Autodesk Inventor part; units mm, degrees
ref_plane "YZ Plane" through (0, 0, 0) normal (1, 0, 0) x (0, 1, 0)
ref_plane "XZ Plane" through (0, 0, 0) normal (0, 1, 0) x (-1, 0, 0)
ref_plane "XY Plane" through (0, 0, 0) normal (0, 0, 1) x (1, 0, 0)
sketch "Sketch1" plane through (0, 0, 0) normal (0, 1, 0) x (-1, 0, 0)
  arc A0 (24.9, 14.1574) -> (29.1, 14.1574) centre (27, 14.1574) ccw
  line L0 (29.1, 14.1574) -> (29.1, 29.1574)
  arc A1 (29.1, 29.1574) -> (24.9, 29.1574) centre (27, 29.1574) ccw
  line L1 (24.9, 29.1574) -> (24.9, 14.1574)
  arc A2 (-29.1, 14.1574) -> (-24.9, 14.1574) centre (-27, 14.1574) ccw
  line L2 (-24.9, 14.1574) -> (-24.9, 29.1574)
  arc A3 (-24.9, 29.1574) -> (-29.1, 29.1574) centre (-27, 29.1574) ccw
  line L3 (-29.1, 29.1574) -> (-29.1, 14.1574)
  ellipse E0 centre (7.3196, 102.715) end of major axis (13.9835, 105.6762) minor radius 6.4402 (10.2387, 108.9524) -> (7.9784, 109.3033) ccw
  line L4 (7.9784, 109.3033) -> (-7.9784, 109.3033)
  ellipse E1 centre (-7.3196, 102.715) end of major axis (-0.6557, 99.7539) minor radius 6.4402 (-7.9784, 109.3033) -> (-10.2387, 108.9524) ccw
  arc A4 (-14.0587, 108.0035) -> (-10.2387, 108.9524) centre (-18.8823, 135.5849) ccw
  arc A5 (-14.0587, 108.0035) -> (-17.7444, 104.1628) centre (-13.2835, 103.5708) ccw
  arc A6 (-18.815, 99.3694) -> (-17.7444, 104.1628) centre (-45.5011, 107.8461) ccw
  line L5 (-18.815, 99.3694) -> (-24.7592, 80.6562)
  arc A7 (-24.7592, 80.6562) -> (-24.9, 79.748) centre (-21.9, 79.748) ccw
  line L6 (-24.9, 79.748) -> (-24.9, 68.8185)
  arc A8 (-27.8412, 67.0538) -> (-24.9, 68.8185) centre (-26.9, 68.8185) ccw
  arc A9 (-27.8412, 67.0538) -> (-30.3028, 66.5886) centre (-28.7824, 65.2891) ccw
  arc A10 (-34.9925, 63.1171) -> (-30.3028, 66.5886) centre (-40.1848, 75.0352) ccw
  arc A11 (-34.9925, 63.1171) -> (-38.8388, 42.8186) centre (-30, 51.6574) ccw
  line L7 (-38.8388, 42.8186) -> (-36.3934, 40.3732)
  arc A12 (-32, 29.7666) -> (-36.3934, 40.3732) centre (-47, 29.7666) ccw
  line L8 (-32, 29.7666) -> (-32, 13.5483)
  arc A13 (-36.3934, 2.9417) -> (-32, 13.5483) centre (-47, 13.5483) ccw
  line L9 (-36.3934, 2.9417) -> (-38.8388, 0.4963)
  arc A14 (-38.8388, 0.4963) -> (-21.1612, -17.1814) centre (-30, -8.3426) ccw
  line L10 (-21.1612, -17.1814) -> (-16.7678, -12.788)
  arc A15 (-12.585, -13.9095) -> (-16.7678, -12.788) centre (-15, -14.5558) ccw
  arc A16 (-12.585, -13.9095) -> (-10.653, -15.3925) centre (-10.653, -13.3925) ccw
  line L11 (-10.653, -15.3925) -> (-8.873, -15.3925)
  arc A17 (-6.9365, -16.8925) -> (-8.873, -15.3925) centre (-8.873, -17.3925) ccw
  arc A18 (-6.9365, -16.8925) -> (-5, -18.3925) centre (-5, -16.3925) ccw
  line L12 (-5, -18.3925) -> (5.127, -18.3925)
  arc A19 (5.127, -18.3925) -> (7.0635, -16.8925) centre (5.127, -16.3925) ccw
  arc A20 (9, -15.3925) -> (7.0635, -16.8925) centre (9, -17.3925) ccw
  line L13 (9, -15.3925) -> (10.653, -15.3925)
  arc A21 (10.653, -15.3925) -> (12.585, -13.9095) centre (10.653, -13.3925) ccw
  arc A22 (16.7678, -12.788) -> (12.585, -13.9095) centre (15, -14.5558) ccw
  line L14 (16.7678, -12.788) -> (21.1612, -17.1814)
  arc A23 (21.1612, -17.1814) -> (38.8387, 0.4964) centre (30, -8.3426) ccw
  line L15 (38.8387, 0.4964) -> (36.3934, 2.9417)
  arc A24 (32, 13.5483) -> (36.3934, 2.9417) centre (47, 13.5483) ccw
  line L16 (32, 13.5483) -> (32, 29.7666)
  arc A25 (36.3934, 40.3732) -> (32, 29.7666) centre (47, 29.7666) ccw
  line L17 (36.3934, 40.3732) -> (38.8388, 42.8186)
  arc A26 (38.8388, 42.8186) -> (34.9925, 63.1171) centre (30, 51.6574) ccw
  arc A27 (30.1775, 66.7374) -> (34.9925, 63.1171) centre (40.1848, 75.0352) ccw
  arc A28 (30.1775, 66.7374) -> (27.769, 67.2622) centre (28.6379, 65.4608) ccw
  arc A29 (24.9, 69.0635) -> (27.769, 67.2622) centre (26.9, 69.0635) ccw
  line L18 (24.9, 69.0635) -> (24.9, 79.748)
  arc A30 (24.9, 79.748) -> (24.7592, 80.6562) centre (21.9, 79.748) ccw
  line L19 (24.7592, 80.6562) -> (18.815, 99.3694)
  arc A31 (17.7444, 104.1628) -> (18.815, 99.3694) centre (45.5011, 107.8461) ccw
  arc A32 (17.7444, 104.1628) -> (14.0587, 108.0035) centre (13.2835, 103.5708) ccw
  arc A33 (10.2387, 108.9524) -> (14.0587, 108.0035) centre (18.8823, 135.5849) ccw
  circle A34 centre (-15.25, 6.4074) radius 3.05
  circle A35 centre (15.25, 36.9074) radius 3.05
  circle A36 centre (15.25, 6.4074) radius 3.05
  circle A37 centre (-15.25, 36.9074) radius 3.05
  circle A38 centre (-18.0312, 75.6574) radius 3
  circle A39 centre (0, 57.6262) radius 3
  circle A40 centre (18.0312, 75.6574) radius 3
  circle A41 centre (0, 93.6886) radius 3
  circle A42 centre (-25.4558, 4.6869) radius 1.55
  circle A43 centre (-13.2835, 103.5708) radius 1.55
  circle A44 centre (-30, -8.3426) radius 1.55
  circle A45 centre (-16.9706, 47.1133) radius 1.55
  circle A46 centre (25.4558, 38.628) radius 1.55
  circle A47 centre (-10, 85.6574) radius 3
  circle A48 centre (30, 51.6574) radius 1.55
  circle A49 centre (-16.9706, -3.7984) radius 1.55
  circle A50 centre (-25.4558, 38.628) radius 1.55
  circle A51 centre (16.9706, 47.1133) radius 1.55
  circle A52 centre (13.2835, 103.5708) radius 1.55
  circle A53 centre (0, 0) radius 1.55
  circle A54 centre (25.4558, 4.6869) radius 1.55
  circle A55 centre (16.9706, -3.7984) radius 1.55
  circle A56 centre (30, -8.3426) radius 1.55
  circle A57 centre (-15.25, 90.9074) radius 3
  circle A58 centre (-10, 65.6574) radius 3
  circle A59 centre (-15.25, 60.4074) radius 3
  circle A60 centre (10, 65.6574) radius 3
  circle A61 centre (15.25, 60.4074) radius 3
  circle A62 centre (-30, 51.6574) radius 1.55
  circle A63 centre (10, 85.6574) radius 3
  circle A64 centre (15.25, 90.9074) radius 3
  point P0 (38.8387, 0.4964)
  point P1 (38.8388, 42.8186)
  point P2 (34.9925, 63.1171)
  point P3 (30.1775, 66.7374)
  point P4 (24.7592, 80.6562)
  point P5 (18.815, 99.3694)
  point P6 (17.7444, 104.1628)
  point P7 (-7.9784, 109.3033)
  point P8 (-10.2387, 108.9524)
  point P9 (-17.7444, 104.1628)
  point P10 (-27.8412, 67.0538)
  point P11 (-30.3028, 66.5886)
  point P12 (-36.3934, 2.9417)
  point P13 (-21.1612, -17.1814)
  point P14 (-12.585, -13.9095)
  point P15 (-6.9365, -16.8925)
  point P16 (7.0635, -16.8925)
  point P17 (29.1, 29.1574)
  point P18 (24.9, 29.1574)
extrude "Extrusion1" add sketch "Sketch1" along normal blind 3
properties part number "Kauri bottom plate V2"
Model file for the job. Use its own axes, mm. A direction names the side the tool comes from. Give positions to 0.01 mm unless a question says otherwise; leave off trailing zeros. Order: outer loops, then holes, each group sorted by start corner. A loop starts at its lowest first (then second) coordinate and runs counter-clockwise, first axis right, second up. Notation, with made-up numbers: (73, -27.5) - (112, -27.5) arc R25 ccw to (112, -14.5) - close; hole circle Ø10 at (-9.75, 24). An arc over 180 degrees is marked (long way). One line per item, written item: value.
Item 1: Tool access for faces 1 (the flat face through (32, 1, 22)), 2 (the flat face through (-18.93, 1.48, -14.95)), 3 (the cylindrical face through (-33.1, 1.5, 35.4)), 4 (the cylindrical face through (15.641, 1.479, 57.433)): list every direction of +Z, -Z, +X, -X, +Y, -Y with a clear straight run to the whole face (end or side of a thin tool).
Response values:
face 1: +X, +Y, -Y
face 2: -Z, +Y, -Y
face 3: -X, +Y, -Y
face 4: +Y, -Y
Item 2: Slice it at C-C (y = 1.5). Give the number of separate pieces and of enclosed holes in the cut face, then the cut area to 3 significant figures.
Response values:
separate pieces: 1
enclosed holes: 33
area: 7,320 mm2
Item 3: Slice it at A-A (x = 0). List the corners of the cut face in (y, z), then the cut area to 3 significant figures.
Response values:
outline: (0, -18.39) - (3, -18.39) - (3, -1.55) - (0, -1.55) - close; (0, 1.55) - (3, 1.55) - (3, 54.63) - (0, 54.63) - close; (0, 60.63) - (3, 60.63) - (3, 90.69) - (0, 90.69) - close; (0, 96.69) - (3, 96.69) - (3, 109.3) - (0, 109.3) - close
area: 338 mm2
Item 4: Wall check: line 1 (Z direction, x = 0, y = 2.2); line 2 (X direction, y = 0.2, z = 76); line 3 (X direction, y = 1.3, z = 21). Give the ranges that are in metal, low to high.
Response values:
line 1: -18.39 to -1.55, 1.55 to 54.63, 60.63 to 90.69, 96.69 to 109.3
line 2: -24.9 to -21.01, -15.05 to 15.05, 21.01 to 24.9
line 3: -32 to -29.1, -24.9 to 24.9, 29.1 to 32
Item 5: Slice it at B-B (z = 23). List the corners of the cut face in (x, y).
Response values:
outline: (-32, 0) - (-29.1, 0) - (-29.1, 3) - (-32, 3) - close; (-24.9, 0) - (24.9, 0) - (24.9, 3) - (-24.9, 3) - close; (29.1, 0) - (32, 0) - (32, 3) - (29.1, 3) - close
Item 6: Pin check, flat tips, straight feed: pin 1 Ø0.9 at (y, z) = (2, 20.5) entering from +X; pin 2 Ø1.9 at (x, z) = (-30, -8.34) entering from +Y; pin 3 Ø3.5 at (x, z) = (25.46, 4.69) entering from -Y. Stop position of each tip, or through.
Response values:
pin 1: x = 32
pin 2: through
pin 3: y = 0
